Build history of the part. All positions in model axes, mm. A direction names the side the tool comes from. Give positions to 0.01 mm unless a question says otherwise; leave off trailing zeros. Order: outer loops, then holes, each group sorted by start corner. A loop starts at its lowest first (then second) coordinate and runs counter-clockwise, first axis right, second up. Notation, with made-up numbers: (-3, -40) - (26, -40) arc R22 cw to (26, -34) - close; hole circle Ø4 at (73, -29). An arc over 180 degrees is marked (long way). Write each question's results on one line, items separated by ' | '. Start each with the question number.
1) Cut at B-B on y = 17. List the corners of the cut face in (x, z), plus the area to 3 significant figures.
2) Drill centre lines: line 1 along Y through (x, z) = (16, 39); line 2 along Z through (x, y) = (0, 0.65). Where is each one in solid material? Low to high. Write a range as from..to.
3) Cut at D-D on y = 8. List the corners of the cut face in (x, z).
4) Cut at A-A on z = 40. List the corners of the cut face in (x, y), plus the area to 3 significant figures.
5) Two-plate mould, pull along Y, no slides. Class faces 6 (the face through (-29.5, 16.9, 1.2)), 7 (the face through (0, 25, 1)), 8 (the face through (0, 14, 0)): +Y half, -Y half, draft (parallel to the pull), parting line (faces both ways), or undercut.
6) Cut at C-C on z = 49. List the corners of the cut face in (x, y), plus the area to 3 significant figures.
7) Drop flat-ended pins along their axis: pin 1 Ø0.8 at (x, z) = (-20.5, 1) entering from -Y; pin 2 Ø1.2 at (y, z) = (1.5, 40.5) entering from +X; pin 3 Ø1.2 at (y, z) = (0.5, 39.5) entering from -X. Give the stop position or say it passes through.
8) Tool access for faces 1 (the face through (-22, 13.5, 1)), 2 (the face through (22, 9, 1)), 3 (the face through (-15.8, 2, 10)), 4 (the face through (-34, 17, 1)), 5 (the face through (20, 1, 40)): list every direction of +Z, -Z, +X, -X, +Y, -Y with a clear straight run to the whole face (end or side of a thin tool).
from build123d import *

# Parameters (mm, degrees)
BOSS_EXTRUDE1_DEPTH       = 2.5
CUT_EXTRUDE1_DEPTH        = 3.5
CUT_EXTRUDE2_DEPTH        = 3.5
SKETCH4_W                 = 31.6
SKETCH4_H                 = 2.5
BOSS_EXTRUDE2_DEPTH       = 22.5
SKETCH5_W                 = 2.5
SKETCH5_H                 = 16
BOSS_EXTRUDE3_DEPTH       = 18.2
SKETCH6_W                 = 2.5
SKETCH6_H                 = 16
BOSS_EXTRUDE4_DEPTH       = 18.2
CUT_EXTRUDE3_DEPTH        = 3.5
CUT_EXTRUDE4_DEPTH        = 61.2
M27_CLEARANCE_HOLE1_D     = 32
M27_CLEARANCE_HOLE1_DEPTH = 2.5
FILLET1_R                 = 2
FILLET2_R                 = 4
FILLET3_R                 = 6


with BuildPart() as part:
    # Sketch1 → Boss-Extrude1 (new body)
    with BuildSketch(Plane(origin=(0, 2.5, 0), x_dir=(1, 0, 0), z_dir=(0, 1, 0))):
        with BuildLine():
            Line((20, -42.835489376), (20, 0))
            Line((20, 0), (-20, 0))
            Line((-20, 0), (-20, -42.835489376))
            ThreePointArc((-20, -42.835489376), (0, -60.2), (20, -42.835489376))
        make_face()
    extrude(amount=-BOSS_EXTRUDE1_DEPTH)

    # Sketch2 → Cut-Extrude1 (cut, through all)
    with BuildSketch(Plane.XZ):
        with BuildLine():
            Line((-15.8, 0), (-15.8, 27.414293822))
            ThreePointArc((-15.8, 27.414293822), (-18.551999405, 32.008547186), (-20, 37.164510624))
            Line((-20, 37.164510624), (-20, 0))
            Line((-20, 0), (-15.8, 0))
        make_face()
    extrude(amount=-CUT_EXTRUDE1_DEPTH, mode=Mode.SUBTRACT)

    # Sketch3 → Cut-Extrude2 (cut, through all)
    with BuildSketch(Plane.XZ):
        with BuildLine():
            Line((20, 0), (20, 37.164510624))
            ThreePointArc((20, 37.164510624), (18.551999405, 32.008547186), (15.8, 27.414293822))
            Line((15.8, 27.414293822), (15.8, 0))
            Line((15.8, 0), (20, 0))
        make_face()
    extrude(amount=-CUT_EXTRUDE2_DEPTH, mode=Mode.SUBTRACT)

    # Sketch4 → Boss-Extrude2 (add)
    with BuildSketch(Plane(origin=(0, 2.5, 0), x_dir=(-1, 0, 0), z_dir=(0, 1, 0))):
        with Locations((0, 1.25)):
            Rectangle(SKETCH4_W, SKETCH4_H)
    extrude(amount=BOSS_EXTRUDE2_DEPTH)

    # Sketch5 → Boss-Extrude3 (add)
    with BuildSketch(Plane(origin=(15.8, 0, 0), x_dir=(0, 0, -1), z_dir=(1, 0, 0))):
        with Locations((-1.25, 17)):
            Rectangle(SKETCH5_W, SKETCH5_H)
    extrude(amount=BOSS_EXTRUDE3_DEPTH)

    # Sketch6 → Boss-Extrude4 (add)
    with BuildSketch(Plane.ZY.offset(15.8)):
        with Locations((1.25, 17)):
            Rectangle(SKETCH6_W, SKETCH6_H)
    extrude(amount=BOSS_EXTRUDE4_DEPTH)

    # Sketch7 → Cut-Extrude3 (cut, through all)
    with BuildSketch(Plane.XY.offset(2.5)):
        with BuildLine():
            Line((26, 20.5), (18, 20.5))
            ThreePointArc((18, 20.5), (14.5, 17), (18, 13.5))
            Line((18, 13.5), (26, 13.5))
            ThreePointArc((26, 13.5), (29.5, 17), (26, 20.5))
        make_face()
    extrude(amount=-CUT_EXTRUDE3_DEPTH, mode=Mode.SUBTRACT)

    # Sketch8 → Cut-Extrude4 (cut, through all)
    with BuildSketch(Plane(origin=(0, 0, 0), x_dir=(-1, 0, 0), z_dir=(0, 0, -1))):
        with BuildLine():
            Line((26, 20.5), (18, 20.5))
            ThreePointArc((18, 20.5), (14.5, 17), (18, 13.5))
            Line((18, 13.5), (26, 13.5))
            ThreePointArc((26, 13.5), (29.5, 17), (26, 20.5))
        make_face()
    extrude(amount=-CUT_EXTRUDE4_DEPTH, mode=Mode.SUBTRACT)

    # M27 Clearance Hole1
    with Locations(Plane(origin=(0, 2.5, 0), x_dir=(1, 0, 0), z_dir=(0, 1, 0))):
        with Locations((0, -40)):
            Hole(M27_CLEARANCE_HOLE1_D / 2, depth=M27_CLEARANCE_HOLE1_DEPTH)

    # Fillet1
    fillet1_edges = [part.edges().sort_by_distance(p)[0] for p in [
        (0, 2.5, 2.5),
    ]]
    fillet(fillet1_edges, radius=FILLET1_R)

    # Fillet2
    fillet2_edges = [part.edges().sort_by_distance(p)[0] for p in [
        (0, 0, 0),
    ]]
    fillet(fillet2_edges, radius=FILLET2_R)

    # Fillet3
    fillet3_edges = [part.edges().sort_by_distance(p)[0] for p in [
        (34, 25, 1.25),
        (34, 9, 1.25),
        (-34, 9, 1.25),
        (-34, 25, 1.25),
    ]]
    fillet(fillet3_edges, radius=FILLET3_R)


solid = part.part
Results:
1) outline: (-34, 0) - (-29.5, 0) - (-29.5, 2.5) - (-34, 2.5) - close; (-14.5, 0) - (14.5, 0) - (14.5, 2.5) - (-14.5, 2.5) - close; (29.5, 0) - (34, 0) - (34, 2.5) - (29.5, 2.5) - close | area: 95.0 mm^2
2) line 1: 0..2.5 | line 2: 1.81..24, 56..60.2
3) outline: (-15.8, 0) - (15.8, 0) - (15.8, 2.5) - (-15.8, 2.5) - close
4) outline: (-20, 0) - (-16, 0) - (-16, 2.5) - (-20, 2.5) - close; (16, 0) - (20, 0) - (20, 2.5) - (16, 2.5) - close | area: 20.0 mm^2
5) face 6: undercut | face 7: +Y half | face 8: draft
6) outline: (-18.08, 0) - (-13.23, 0) - (-13.23, 2.5) - (-18.08, 2.5) - close; (13.23, 0) - (18.08, 0) - (18.08, 2.5) - (13.23, 2.5) - close | area: 24.3 mm^2
7) pin 1: y = 9 | pin 2: x = 20 | pin 3: x = -20
8) face 1: +Z, -Z | face 2: +Z, -Z, +X, -Y | face 3: -Z, -X, -Y | face 4: +Z, -Z, -X, +Y, -Y | face 5: +Z, -Z, +X, +Y, -Y
